Could you check a few things on this model? Use its own coordinates, in mm. Coordinates: 2 decimals unless noted, no trailing zeros. Order: outer loops, then holes, each group sorted by start corner. A loop starts at its lowest first (then second) coordinate and runs counter-clockwise, first axis right, second up. Notation, with made-up numbers: (42, 33) - (84, 33) arc R15 ccw to (84, 58) - close; hole circle Ø10 at (39, 76). An arc over 180 degrees is marked (long way). Answer as CSV lines item,"result". Start each with the question number.
1. I want a section at C-C, the plane z = 102. List the corners of the cut face in (x, y) for me, and give its area (3 significant figures).
2. I want a section at B-B, the plane y = -9.5. Count the separate pieces of the cut face and the enclosed holes in it, and give its area (3 significant figures).
3. For pin 1 (1 mm diameter, centred on y = -9.5, z = -2.5, fed in from +X); pin 2 (5 mm diameter, centred on x = 0, y = -3, fed in from +Z); pin 3 (4 mm diameter, centred on x = -69.42, z = 17.11, fed in from +Y), each with a flat end and sliding along its axis, tell me the tip position at first contact or that it passes through.
4. I want a section at A-A, the plane x = 16.5. List the corners of the cut face in (y, z) for me, and give its area (3 significant figures).
5. Thinking about a two-plate mould opening in Z: for faces 1 (the face through (-90.468, -6.268, -93.528)), 2 (the face through (-89, -6, 92)), 3 (the face through (-25, -12.7, 21)), which applies, released by +Z, released by -Z, zero draft, split by the parting line, or undercut?
6. I need wall thicknesses on probe 1 along X at (y, z) = (-7, 38); probe 2 along Z at (x, y) = (-88.5, -0.75); probe 3 along X at (y, z) = (-5.25, -60). Which ranges of each line are inside material? Lowest first, please.
from build123d import *

# Parameters (mm, degrees)
F0_R     = 3.302
F0_R_2   = 1.7
F0_R_3   = 18
F1_DEPTH = 12.7
F2_R     = 5.08
F3_SIZE  = 0.508


with BuildPart() as f1:
    # F0 (on Front) → F1 (new body)
    with BuildSketch(Plane.XZ):
        with BuildLine():
            Line((108.426517, -114.299545), (0.476517, 152.400455))
            Line((0.476517, 152.400455), (-107.473483, 152.400455))
            Line((-107.473483, 152.400455), (-107.473483, -76.199545))
            ThreePointArc((-107.473483, -76.199545), (-90.99167, -92.728336), (-82.073483, -114.299545))
            Line((-82.073483, -114.299545), (108.426517, -114.299545))
        make_face()
        with Locations((-88.423483, -57.137189)):
            Circle(F0_R, mode=Mode.SUBTRACT)
        with Locations((-88.423483, -19.037189)):
            Circle(F0_R, mode=Mode.SUBTRACT)
        with Locations((-92.919483, 14.618093)):
            Circle(F0_R_2, mode=Mode.SUBTRACT)
        with Locations((-69.424483, 17.113093)):
            Circle(F0_R_2, mode=Mode.SUBTRACT)
        with Locations((-45.929483, 14.618093)):
            Circle(F0_R_2, mode=Mode.SUBTRACT)
        with Locations((-90.424483, 38.113093)):
            Circle(F0_R_2, mode=Mode.SUBTRACT)
        with Locations((-69.424483, 38.113093)):
            Circle(F0_R_3, mode=Mode.SUBTRACT)
        with Locations((-92.919483, 61.608093)):
            Circle(F0_R_2, mode=Mode.SUBTRACT)
        with Locations((-69.424483, 59.113093)):
            Circle(F0_R_2, mode=Mode.SUBTRACT)
        with Locations((-48.424483, 38.113093)):
            Circle(F0_R_2, mode=Mode.SUBTRACT)
        with Locations((-45.929483, 61.608093)):
            Circle(F0_R_2, mode=Mode.SUBTRACT)
        with Locations((-88.423483, 95.250455)):
            Circle(F0_R, mode=Mode.SUBTRACT)
        with Locations((-88.423483, 133.350455)):
            Circle(F0_R, mode=Mode.SUBTRACT)
        with Locations((-92.919483, 14.618093)):
            Circle(F0_R_2)
        with Locations((-45.929483, 14.618093)):
            Circle(F0_R_2)
        with Locations((-45.929483, 61.608093)):
            Circle(F0_R_2)
        with Locations((-92.919483, 61.608093)):
            Circle(F0_R_2)
    extrude(amount=F1_DEPTH)

    # F2
    f2_edges = [f1.edges().sort_by_distance(p)[0] for p in [
        (-107.473483, -6.35, 152.400455),
        (0.476517, -6.35, 152.400455),
        (-107.473483, -6.35, -76.199545),
    ]]
    fillet(f2_edges, radius=F2_R)

    # F3
    f3_edges = [f1.edges().sort_by_distance(p)[0] for p in [
        (55.093878, -12.7, 17.463445),
        (-0.108282, -12.7, 151.532864),
        (13.176517, -12.7, -114.299545),
        (-52.670567, -12.7, 152.400455),
        (-90.299941, -12.7, -93.790077),
        (-105.985585, -12.7, 150.912558),
        (-106.925335, -12.7, -75.855453),
        (-107.473483, -12.7, 36.880185),
        (-91.725483, -12.7, -57.137189),
        (-91.725483, -12.7, -19.037189),
        (-71.124483, -12.7, 17.113093),
        (-92.124483, -12.7, 38.113093),
        (-87.424483, -12.7, 38.113093),
        (-71.124483, -12.7, 59.113093),
        (-50.124483, -12.7, 38.113093),
        (-91.725483, -12.7, 95.250455),
        (-91.725483, -12.7, 133.350455),
        (55.093878, 0, 17.463445),
        (-0.108282, 0, 151.532864),
        (13.176517, 0, -114.299545),
        (-52.670567, 0, 152.400455),
        (-90.299941, 0, -93.790077),
        (-105.985585, 0, 150.912558),
        (-106.925335, 0, -75.855453),
        (-107.473483, 0, 36.880185),
        (-91.725483, 0, -57.137189),
        (-91.725483, 0, -19.037189),
        (-71.124483, 0, 17.113093),
        (-92.124483, 0, 38.113093),
        (-87.424483, 0, 38.113093),
        (-71.124483, 0, 59.113093),
        (-50.124483, 0, 38.113093),
        (-91.725483, 0, 95.250455),
        (-91.725483, 0, 133.350455),
    ]]
    chamfer(f3_edges, length=F3_SIZE)


solid = f1.part
Solved:
1,outline,"(-107.47, -12.19) - (-106.97, -12.7) - (20.33, -12.7) - (20.88, -12.19) - (20.88, -0.51) - (20.33, 0) - (-106.97, 0) - (-107.47, -0.51) - close"
1,area,"1,630 mm2"
2,separate pieces,"1"
2,enclosed holes,"9"
2,area,"41,400 mm2"
3,pin 1,"stops at x = 63.38"
3,pin 2,"stops at z = 152.38"
3,pin 3,"stops at y = -0.2"
4,outline,"(-12.7, -113.79) - (-12.19, -114.3) - (-0.51, -114.3) - (0, -113.79) - (0, 111.46) - (-0.51, 112.81) - (-12.19, 112.81) - (-12.7, 111.46) - close"
4,area,"2,880 mm2"
5,face 1,"released by -Z"
5,face 2,"undercut"
5,face 3,"zero draft"
6,probe 1,"x = -107.47 to -92.12, -88.73 to -87.42, -51.42 to -50.12, -46.73 to 46.78"
6,probe 2,"z = -96.81 to -60.44, -53.84 to -22.34, -15.74 to 91.95, 98.55 to 130.05, 136.65 to 152.4"
6,probe 3,"x = -107.47 to -90.07, -86.78 to 86.45"
